```python
from build123d import *

# Parameters (mm, degrees)
SKETCH1_W             = 38
SKETCH1_H             = 52
EXTRUDE1_DEPTH        = 15
SKETCH4_W             = 38
SKETCH4_H             = 26
CUT_EXTRUDE3_DEPTH    = 16
F_8_CLEARANCE_HOLE2_D = 4.4958


with BuildPart() as part:
    # Sketch1 → Extrude1 (new body)
    with BuildSketch(Plane.XY):
        with Locations((0, 26)):
            Rectangle(SKETCH1_W, SKETCH1_H)
    extrude(amount=EXTRUDE1_DEPTH)

    # Sketch4 → Cut-Extrude3 (cut, through all)
    with BuildSketch(Plane.XY.offset(15)):
        with Locations((0, 39)):
            Rectangle(SKETCH4_W, SKETCH4_H)
    extrude(amount=-CUT_EXTRUDE3_DEPTH, mode=Mode.SUBTRACT)

    # #8 Clearance Hole2 (through all)
    with Locations(Plane(origin=(0, 26, 0), x_dir=(-1, 0, 0), z_dir=(0, 1, 0))):
        with Locations((-4.7625, 6.35), (4.7625, 6.35)):
            Hole(F_8_CLEARANCE_HOLE2_D / 2)


solid = part.part
```
CAD build for the part. Positions are in the model's coordinates, mm. Coordinates: 2 decimals unless noted, no trailing zeros. Write each loop counter-clockwise with the first axis right and the second up, starting at its lowest first coordinate (ties: lowest second). Pieces come first, ordered by that corner, then holes. Notation, with made-up numbers: (79.5, -9) -> (115.5, -9) arc R17 ccw to (115.5, -2) -> close; hole circle Ø11 at (-26, 29.5). An arc over 180 degrees is marked (long way). Return JSON: item names as keys, results as strings. Group by question number.
Q1. Cut at A-A, the plane z = 6.35. Give the cut face in (x, y), then the cut area to 3 significant figures.
Q2. Cut at C-C, the plane y = 12.75. Give the cut face in (x, z), then the cut area to 3 significant figures.
Q3. Flat gauge pin, fed straight in: pin 1 (2 mm diameter, centred on x = 13.5, y = 21, fed in from -Z). Where does the tip first touch, or does it go through?
Q4. Drill centre lines: line 1 (X direction, y = 8.5, z = 6.25); line 2 (X direction, y = 22.5, z = 8.25). Where is each one in solid material? Low to high.
Q5. Pull direction X, two halves, no side cores. Call faces 1 (the face through (19, 13, 7)), 2 (the face through (-6.42, 12.82, 7.87)), 3 (the face through (0, 26, 8)): released by +X, released by -X, zero draft, split by the parting line, or undercut.
Q6. Cut at B-B, the plane x = -5. Give the cut face in (y, z), then the cut area to 3 significant figures.
Returned:
{
 "1": {"outline": "(-19, 0) -> (-7.01, 0) -> (-7.01, 26) -> (-19, 26) -> close; (-2.51, 0) -> (2.51, 0) -> (2.51, 26) -> (-2.51, 26) -> close; (7.01, 0) -> (19, 0) -> (19, 26) -> (7.01, 26) -> close", "area": "754 mm2"},
 "2": {"outline": "(-19, 0) -> (19, 0) -> (19, 15) -> (-19, 15) -> close; hole circle Ø4.5 at (-4.76, 6.35); hole circle Ø4.5 at (4.76, 6.35)", "area": "538 mm2"},
 "3": {"pin 1": "stops at z = 0"},
 "4": {"line 1": "x = -19 to -7.01, -2.52 to 2.52, 7.01 to 19", "line 2": "x = -19 to -5.96, -3.56 to 3.56, 5.96 to 19"},
 "5": {"face 1": "released by +X", "face 2": "undercut", "face 3": "zero draft"},
 "6": {"outline": "(0, 0) -> (26, 0) -> (26, 4.11) -> (0, 4.11) -> close; (0, 8.59) -> (26, 8.59) -> (26, 15) -> (0, 15) -> close", "area": "274 mm2"}
}
